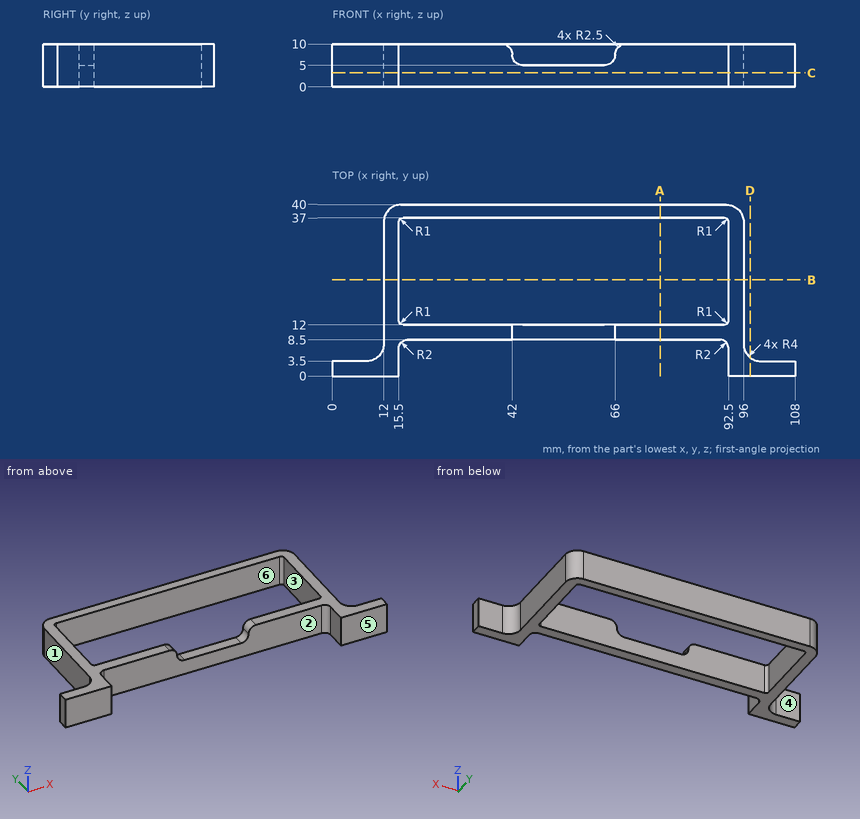
Can you work these out from the drawing? Everything is in mm from the part's minimum corner. A direction names the side the tool comes from. Give positions to 0.01 mm unless a question says otherwise; leave off trailing zeros. Order: outer loops, then holes, each group sorted by start corner. A loop starts at its lowest first (then second) coordinate and runs counter-clockwise, first axis right, second up.
1. I need wall thicknesses on L1, parallel to X at y = 19.5, z = 6.75; L2, parallel to Y at x = 57.5, z = 3.5; L3, parallel to Z at x = 48.5, y = 11. Which ranges of each line are inside material? Lowest first, please.
2. We'd pull the mould along Y, two halves only. Please class the marked faces 4, 5 and 6: pulls with the +Y half, pulls with the -Y half, needs draft (parallel to the pull), parting line crosses it, or undercut.
3. Suppose I cut it at C-C (z = 3.25). List the corners of the cut face in (x, y) for me, plus the area to 3 significant figures.
4. Suppose I cut it at D-D (x = 97.5). List the corners of the cut face in (y, z) for me, plus the area to 3 significant figures.
5. Will these pins go through, and if not, where does the flat tip stop? P1, Ø3, axis at x = 51.5, y = 11, coming from the +Z side; P2, Ø2.5, axis at x = 102.5, z = 4, coming from the +Y side; P3, Ø5, axis at y = 22, z = 6, coming from the -X side.
6. Suppose I cut it at B-B (y = 22.5). List the corners of the cut face in (x, z) for me.
7. For the marked faces 1, 2 and 3, which set-ups out of +Z, -Z, +X, -X, +Y, -Y let a thin tool reach every point of the face, with its end or its side?
8. Suppose I cut it at A-A (x = 76.5). List the corners of the cut face in (y, z) for me.
Solved:
1. L1: x = 12 to 15.5, 92.5 to 96
1. L2: y = 8.5 to 12, 37 to 40
1. L3: z = 0 to 5
2. face 4: pulls with the +Y half
2. face 5: pulls with the -Y half
2. face 6: undercut
3. outline: (0, 0) - (15.5, 0) - (15.5, 6.5) arc R2 cw to (17.5, 8.5) - (90.5, 8.5) arc R2 cw to (92.5, 6.5) - (92.5, 0) - (108, 0) - (108, 3.5) - (100, 3.5) arc R4 cw to (96, 7.5) - (96, 36) arc R4 ccw to (92, 40) - (16, 40) arc R4 ccw to (12, 36) - (12, 7.5) arc R4 cw to (8, 3.5) - (0, 3.5) - close; hole (15.5, 13) arc R1 ccw to (16.5, 12) - (91.5, 12) arc R1 ccw to (92.5, 13) - (92.5, 36) arc R1 ccw to (91.5, 37) - (16.5, 37) arc R1 ccw to (15.5, 36) - close
3. area: 867 mm2
4. outline: (0, 0) - (4.38, 0) - (4.38, 10) - (0, 10) - close
4. area: 43.8 mm2
5. P1: stops at z = 5
5. P2: stops at y = 3.5
5. P3: stops at x = 12
6. outline: (12, 0) - (15.5, 0) - (15.5, 10) - (12, 10) - close; (92.5, 0) - (96, 0) - (96, 10) - (92.5, 10) - close
7. face 1: +Z, -Z, -X, +Y
7. face 2: +Z, -Z, -Y
7. face 3: +Z, -Z
8. outline: (8.5, 0) - (12, 0) - (12, 10) - (8.5, 10) - close; (37, 0) - (40, 0) - (40, 10) - (37, 10) - close
